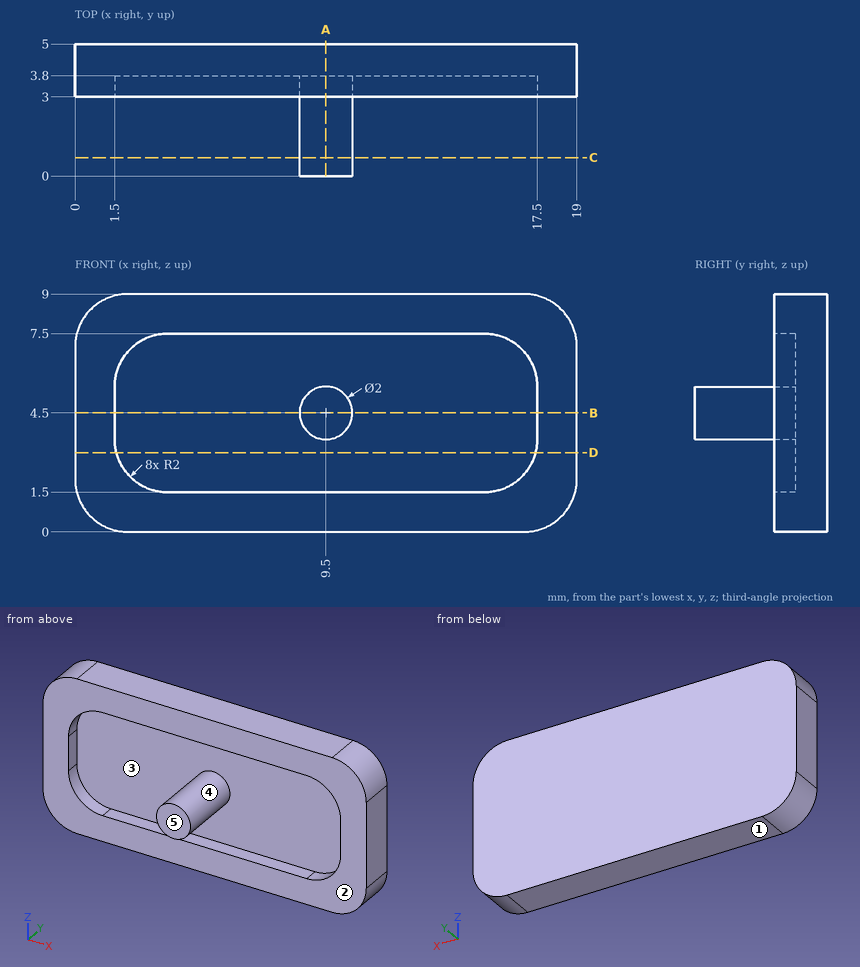
Geometry check sheet. Reference: drawing and pictorial views, mm from the part's lowest x, y, z. A direction names the side the tool comes from. Round coordinates to 2 decimals unless told otherwise and drop trailing zeros. Write each loop counter-clockwise with the first axis right and the second up, starting at its lowest first coordinate (ties: lowest second). Pieces come first, ordered by that corner, then holes. Notation, with made-up numbers: (36, -16.5) -> (81, -16.5) arc R24 ccw to (81, 13.5) -> close; hole circle Ø5 at (85, -10.75). An arc over 180 degrees is marked (long way). Answer as CSV lines item,"result". Start each with the question number.
1) Material ranges on line 1 (Y direction, x = 6, z = 5.25); line 2 (Y direction, x = 1.5, z = 7); line 3 (X direction, y = 3.4, z = 8.25), recorded low to high. Write a range as from..to.
2) Section check A-A on x = 9.5. Enter the section's corners in (y, z), and give its area (3 significant figures).
3) Tool access check on the marked faces 4 and 5. Record the directions out of +Z, -Z, +X, -X, +Y, -Y that give a thin tool (end or side, any length) a straight path to the whole face; none if there is none.
4) Section check D-D on z = 3. Enter the section's corners in (x, y).
5) Section check B-B on z = 4.5. Enter the section's corners in (x, y).
6) Release check for a two-part mould opening along Z. For the marked faces 1, 2 and 3 record: pulls with the +Z half, pulls with the -Z half, needs draft (parallel to the pull), parting line crosses it, or undercut.
7) Go/stop test with flat-tipped pins: P1, Ø2.5, axis at x = 13.5, z = 4.5, coming from the -Y side; P2, Ø1.8, axis at x = 9.5, z = 3, coming from the -Y side. Record where each tip stops, or that it passes through.
8) Section check C-C on y = 0.7. Enter the section's corners in (x, z), and give its area (3 significant figures).
Found:
1,line 1,"y = 3.8..5"
1,line 2,"y = 3..5"
1,line 3,"x = 0.44..18.56"
2,outline,"(0, 3.5) -> (3.8, 3.5) -> (3.8, 1.5) -> (3, 1.5) -> (3, 0) -> (5, 0) -> (5, 9) -> (3, 9) -> (3, 7.5) -> (3.8, 7.5) -> (3.8, 5.5) -> (0, 5.5) -> close"
2,area,"20.8 mm^2"
3,face 4,"-Y"
3,face 5,"+Z, -Z, +X, -X, -Y"
4,outline,"(0, 3) -> (1.56, 3) -> (1.56, 3.8) -> (17.44, 3.8) -> (17.44, 3) -> (19, 3) -> (19, 5) -> (0, 5) -> close"
5,outline,"(0, 3) -> (1.5, 3) -> (1.5, 3.8) -> (8.5, 3.8) -> (8.5, 0) -> (10.5, 0) -> (10.5, 3.8) -> (17.5, 3.8) -> (17.5, 3) -> (19, 3) -> (19, 5) -> (0, 5) -> close"
6,face 1,"pulls with the -Z half"
6,face 2,"needs draft"
6,face 3,"undercut"
7,P1,"stops at y = 3.8"
7,P2,"stops at y = 0"
8,outline,"circle Ø2 at (9.5, 4.5)"
8,area,"3.14 mm^2"
